from build123d import *

# Parameters (mm, degrees)
CROQUIS1_R              = 8.35
SALIENTE_EXTRUIR1_DEPTH = 17.5
SALIENTE_EXTRUIR2_DEPTH = 11
CROQUIS4_R              = 8.35
CORTAR_EXTRUIR1_DEPTH   = 55


with BuildPart() as part:
    # Croquis1 → Saliente-Extruir1 (new, symmetric)
    with BuildSketch(Plane.XY):
        with BuildLine():
            Line((-11.35, -15), (11.35, -15))
            Line((11.35, -15), (11.35, 0))
            ThreePointArc((11.35, 0), (0, 11.35), (-11.35, 0))
            Line((-11.35, 0), (-11.35, -15))
        make_face()
        Circle(CROQUIS1_R, mode=Mode.SUBTRACT)
    extrude(amount=SALIENTE_EXTRUIR1_DEPTH, both=True)

    # Croquis2 → Saliente-Extruir2 (add, symmetric)
    with BuildSketch(Plane(origin=(0, 0, 0), x_dir=(0, 0, -1), z_dir=(1, 0, 0))):
        with BuildLine():
            Line((-17.5, -15), (-17.5, -35))
            Line((-17.5, -35), (3.713203436, -56.213203436))
            Line((3.713203436, -56.213203436), (21.390872965, -38.535533906))
            Line((21.390872965, -38.535533906), (4.683766184, -21.828427125))
            ThreePointArc((4.683766184, -21.828427125), (3.816675179, -17.469266271), (7.512193309, -15))
            Line((7.512193309, -15), (-17.5, -15))
        make_face()
    extrude(amount=SALIENTE_EXTRUIR2_DEPTH, both=True)

    # Croquis4 → Cortar-Extruir1 (cut)
    with BuildSketch(Plane(origin=(0, -29.963203436, -29.963203436), x_dir=(-1, 0, 0), z_dir=(0, -0.7071067811865459, -0.7071067811865492))):
        with Locations(Location((0, -24.623106012, 0), (0, 0, 90))):
            Circle(CROQUIS4_R)
    extrude(amount=-CORTAR_EXTRUIR1_DEPTH, mode=Mode.SUBTRACT)


solid = part.part
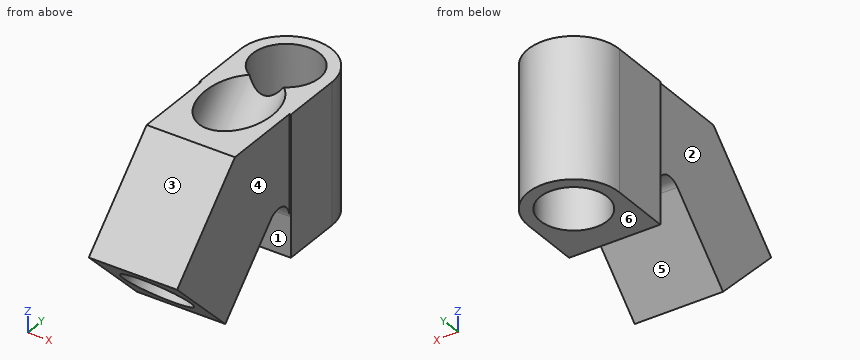
Geometry check sheet. Reference: the model listing, model coordinates, mm. Face numbers are marked on the shaded views. A direction names the side the tool comes from. Round coordinates to 2 decimals unless told otherwise and drop trailing zeros. Loops run counter-clockwise (first coordinate to the right, second up) from the corner with the lowest first, then second, coordinate; pieces in that order, holes last. Notation, with made-up numbers: (15.5, -20.5) -> (60.5, -20.5) arc R25 cw to (60.5, -8.5) -> close; hole circle Ø4 at (-18, 3.25). An arc over 180 degrees is marked (long way). Answer as a JSON object with one key per item and string values. Group by question number.
Item 1: Cross-section at D-D, the plane x = 0. Record the cut outline in (y, z).
Item 2: Cross-section at B-B, the plane y = -4.5. Record the cut outline in (x, z), plus the area to 3 significant figures.
Item 3: Thickness scan on line 1 along Y through (x, z) = (0, 7); line 2 along Y through (x, z) = (0, -1); line 3 along Z through (x, y) = (-8.75, 5). Record the ranges inside material, lowest first.
Item 4: Cross-section at C-C, the plane z = -9. Count the separate pieces of the cut face and the enclosed holes in it, plus the area to 3 significant figures.
Item 5: Release check for a two-part mould opening along Y. For the marked faces 1, 2 and 3 record: pulls with the +Y half, pulls with the -Y half, needs draft (parallel to the pull), parting line crosses it, or undercut.
Item 6: Cross-section at A-A, the plane x = -7.25. Record the cut outline in (y, z).
Item 7: Set-up check for the marked faces 4, 5 and 6: record each of +Z, -Z, +X, -X, +Y, -Y from which the full face is reachable in a straight line by a thin tool's end or side.
Item 8: Depth check by flat-ended pin: pin 1 Ø4 at (x, y) = (-3.5, -35.5) entering from -Z; pin 2 Ø11.5 at (x, y) = (4, 3.5) entering from -Z; pin 3 Ø12 at (x, y) = (6.5, -48) entering from +Z; pin 4 Ø2 at (y, z) = (-46, 10.5) entering from +X. Enter the tip coordinate at first touch or a pass-through.
Determined:
{
 "1": {"outline": "(-56.21, -3.71) -> (-53.28, -6.65) -> (-29.13, 17.5) -> (-35, 17.5) -> close; (-41.47, -18.46) -> (-38.54, -21.39) -> (-21.83, -4.68) arc R4 cw to (-15, -7.51) -> (-15, -17.5) -> (-8.35, -17.5) -> (-8.35, 14.66) -> close; (8.35, -17.5) -> (11.35, -17.5) -> (11.35, 17.5) -> (8.35, 17.5) -> close"},
 "2": {"outline": "(-11.35, -17.5) -> (-7.03, -17.5) -> (-7.03, 17.5) -> (-11.35, 17.5) -> close; (7.03, -17.5) -> (11.35, -17.5) -> (11.35, 17.5) -> (7.03, 17.5) -> close", "area": "302 mm²"},
 "3": {"line 1": "y = -45.5 to -39.63, -16.01 to -8.35, 8.35 to 11.35", "line 2": "y = -53.5 to -47.63, -24.01 to -8.35, 8.35 to 11.35", "line 3": "z = -17.5 to 17.5"},
 "4": {"separate pieces": "2", "enclosed holes": "1", "area": "603 mm²"},
 "5": {"face 1": "undercut", "face 2": "needs draft", "face 3": "pulls with the -Y half"},
 "6": {"outline": "(-56.21, -3.71) -> (-50.3, -9.62) -> (-23.18, 17.5) -> (-35, 17.5) -> close; (-44.45, -15.48) -> (-38.54, -21.39) -> (-21.83, -4.68) arc R4 cw to (-15, -7.51) -> (-15, -17.5) -> (-4.14, -17.5) -> (-4.14, 17.5) -> (-11.46, 17.5) -> close; (4.14, -17.5) -> (8.73, -17.5) -> (8.73, 17.5) -> (4.14, 17.5) -> close"},
 "7": {"face 4": "+Z, -Z, +X, -Y", "face 5": "-Z, +X, -X", "face 6": "-Z, +X, -X, +Y"},
 "8": {"pin 1": "stops at z = -20.36", "pin 2": "stops at z = -17.5", "pin 3": "stops at z = 10.5", "pin 4": "passes through"}
}
